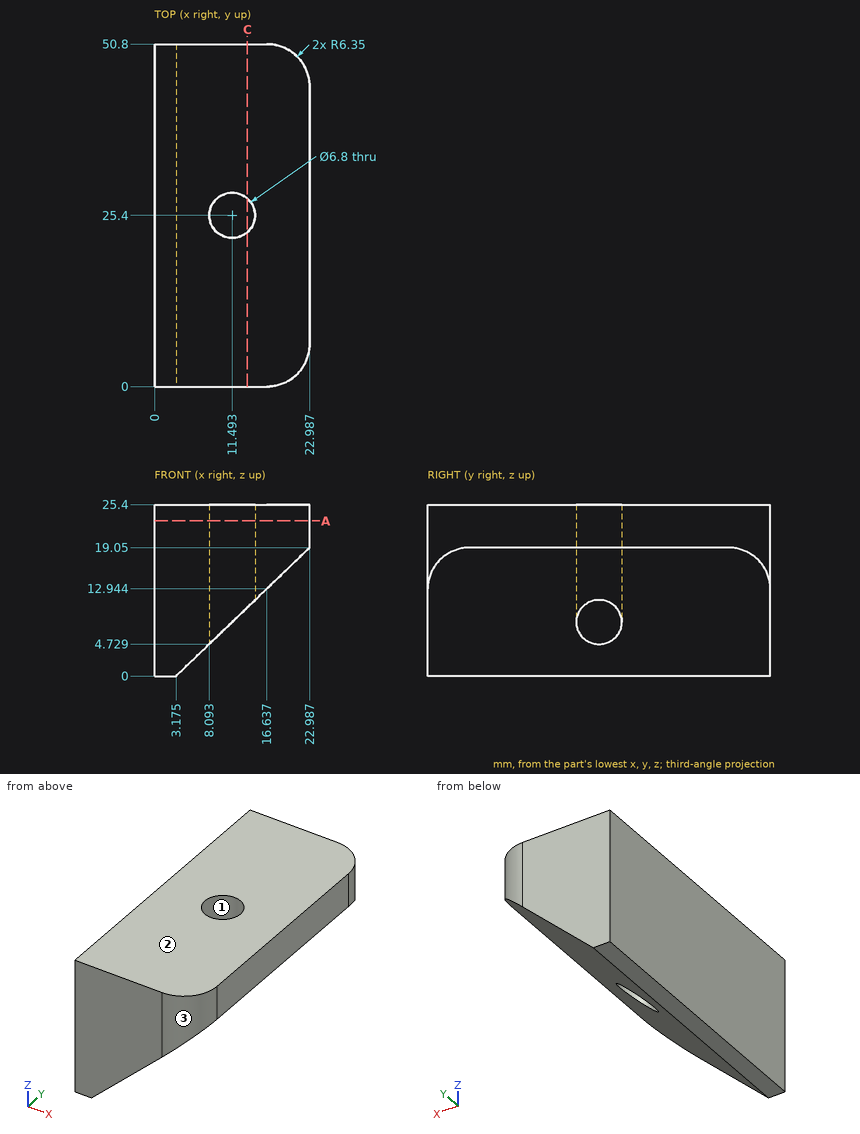
The drawing under review shows one solid part. Ordinate dimensions are in mm from its lowest x, y, z. Round coordinates to 2 decimals unless told otherwise and drop trailing zeros. Loops run counter-clockwise (first coordinate to the right, second up) from the corner with the lowest first, then second, coordinate; pieces in that order, holes last.
Item 1: Take a section at C-C (x = 13.75). Write out the cut boundary in (y, z), then the cut area to 3 significant figures.
Determined:
outline: (0, 10.17) - (22.86, 10.17) - (22.86, 25.4) - (0, 25.4) - close; (27.94, 10.17) - (50.8, 10.17) - (50.8, 25.4) - (27.94, 25.4) - close
area: 696 mm2
Item 2: Mouldability with a two-part tool opening along X and no side actions: class the marked faces 1, 2 and 3 as released by +X, released by -X, zero draft, split by the parting line, or undercut.
Determined:
face 1: undercut
face 2: zero draft
face 3: released by +X
Item 3: Clearance check with flat-ended pins moving along their axes: pin 1 Ø12 at (x, z) = (18, 4) entering from -Y; pin 2 Ø8 at (x, y) = (18.5, 35) entering from -Z; pin 3 Ø1.5 at (x, y) = (17.5, 21) entering from -Z; pin 4 Ø4 at (x, y) = (20.5, 45) entering from -Z (1 decimal). State where each tip first meets the part, or that it passes through.
Determined:
pin 1: passes through
pin 2: stops at z = 10.89
pin 3: stops at z = 13.05
pin 4: stops at z = 14.7
Item 4: Take a section at A-A (z = 23). Write out the cut boundary in (x, y), then the cut area to 3 significant figures.
Determined:
outline: (0, 0) - (16.64, 0) arc R6.35 ccw to (22.99, 6.35) - (22.99, 44.45) arc R6.35 ccw to (16.64, 50.8) - (0, 50.8) - close; hole circle Ø6.8 at (11.49, 25.4)
area: 1,110 mm2
Item 5: For line 1 (Y direction, x = 10.25, z = 14.25) (1 decimal); line 2 (Y direction, x = 9, z = 8.25); line 3 (X direction, y = 25.4, z = 15.5) (1 decimal), list the stretches that pass through material, from the lowest coordinate up.
Determined:
line 1: y = 0 to 22.2, 28.6 to 50.8
line 2: y = 0 to 23.09, 27.71 to 50.8
line 3: x = 0 to 8.1, 14.9 to 19.3
